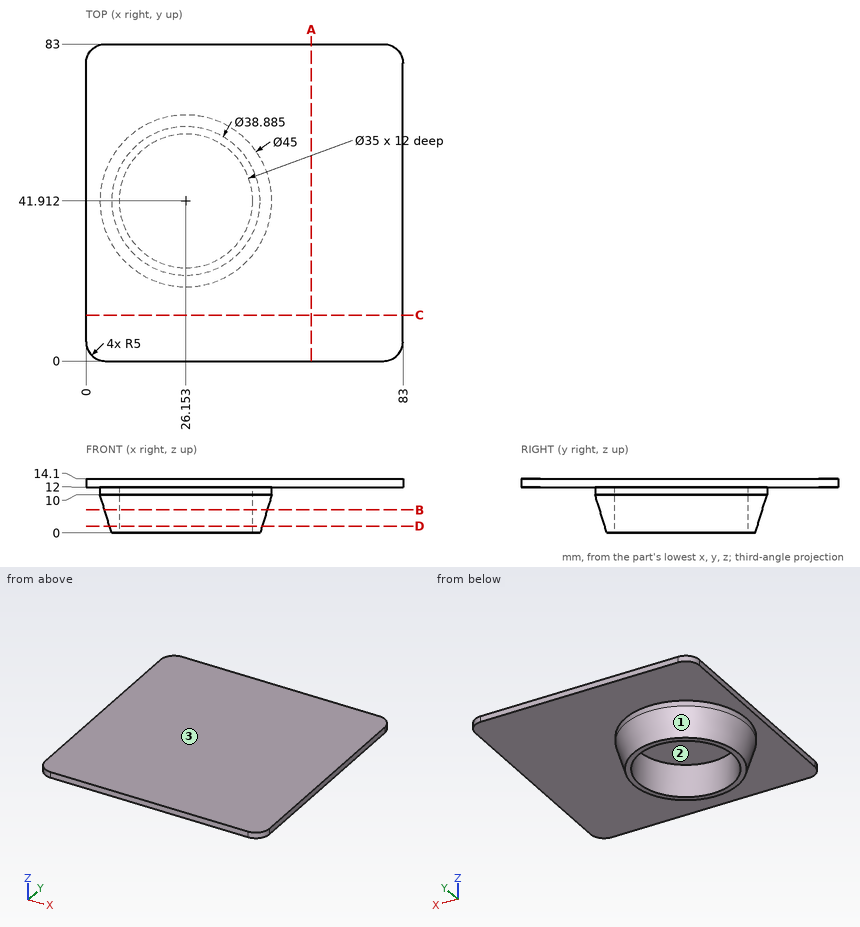
Input: dimensioned drawing with shaded views. Units: mm. Origin: part minimum x, y, z. Round coordinates to 2 decimals unless told otherwise and drop trailing zeros. Loops run counter-clockwise (first coordinate to the right, second up) from the corner with the lowest first, then second, coordinate; pieces in that order, holes last. Notation, with made-up numbers: M 85.5,35.5 L 93.5,35.5 A32 ccw 93.5,63.5 Z; hole C 21,64.5 d11. An arc over 180 degrees is marked long. Return JSON: item names as keys, results as strings. Group by question number.
1. Material intervals for line 1 along Z through (x, y) = (13, 48.5); line 2 along Y through (x, z) = (37.5, 8.75) (1 decimal); line 3 along X through (y, z) = (46, 8.25) (1 decimal), sorted ascending. Write a range as from..to.
2. Section query A-A on x = 59. Output: boundary loops of the cut face in (y, z), and give its area (3 significant figures).
3. Section query D-D on z = 1.75. Output: boundary loops of the cut face in (x, y) (1 decimal), and give its area (3 significant figures).
4. Pin query (flat end, axial travel): pin 1 (3 mm diameter, centred on x = 65.5, y = 16, fed in from -Z); pin 2 (8 mm diameter, centred on x = 26, z = 3, fed in from -Y); pin 3 (5 mm diameter, centred on x = 42.5, z = 2, fed in from -Y). Return the tip coordinate at first contact, or that it passes through.
5. Section query B-B on z = 6. Output: boundary loops of the cut face in (x, y), and give its area (3 significant figures).
6. Mould query, pull axis Y, two halves, no side actions, for the marked faces 1, 2 and 3. Classes: released by +Y, released by -Y, zero draft, split by the parting line, or undercut.
Checks:
{
 "1": {"line 1": "z = 12..14.1", "line 2": "y = 22.9..28.6, 55.2..60.9", "line 3": "x = 4.6..9.1, 43.2..47.7"},
 "2": {"outline": "M 0,12 L 83,12 L 83,14.1 L 0,14.1 Z", "area": "174 mm²"},
 "3": {"outline": "C 26.2,41.9 d40; hole C 26.2,41.9 d35", "area": "292 mm²"},
 "4": {"pin 1": "stops at z = 12", "pin 2": "stops at y = 20.33", "pin 3": "stops at y = 27.18"},
 "5": {"outline": "C 26.15,41.91 d42.55; hole C 26.15,41.91 d35", "area": "460 mm²"},
 "6": {"face 1": "split by the parting line", "face 2": "undercut", "face 3": "zero draft"}
}
